from build123d import *

# Parameters (mm, degrees)
SKETCH1_W           = 8.5
SKETCH1_H           = 20
BOSS_EXTRUDE1_DEPTH = 20
SKETCH4_R           = 1
BOSS_EXTRUDE2_DEPTH = 1.5
SKETCH6_R           = 3
BOSS_EXTRUDE3_DEPTH = 3
SKETCH7_R           = 1.5
BOSS_EXTRUDE4_DEPTH = 4


with BuildPart() as part:
    # Sketch1 → Boss-Extrude1 (new body)
    with BuildSketch(Plane(origin=(0, 0, 0), x_dir=(1, 0, 0), z_dir=(0, 1, 0))):
        Rectangle(SKETCH1_W, SKETCH1_H)
    extrude(amount=BOSS_EXTRUDE1_DEPTH)

    # Sketch4 → Boss-Extrude2 (add)
    with BuildSketch(Plane(origin=(0, 15, 0), x_dir=(1, 0, 0), z_dir=(0, 1, 0))):
        Polygon((-4.25, 10), (4.25, 10), (4.25, 11.75), (2.75, 13.25), (-2.75, 13.25), (-4.25, 11.75), align=None)
        with Locations((0, 11.75)):
            Circle(SKETCH4_R, mode=Mode.SUBTRACT)
        Polygon((-2.75, -13.25), (2.75, -13.25), (4.25, -11.75), (4.25, -10), (-4.25, -10), (-4.25, -11.75), align=None)
        with Locations((0, -11.75)):
            Circle(SKETCH4_R, mode=Mode.SUBTRACT)
    extrude(amount=BOSS_EXTRUDE2_DEPTH)

    # Sketch6 → Boss-Extrude3 (add)
    with BuildSketch(Plane(origin=(0, 20, 0), x_dir=(1, 0, 0), z_dir=(0, 1, 0))):
        with Locations((0, 7)):
            Circle(SKETCH6_R)
    extrude(amount=BOSS_EXTRUDE3_DEPTH)

    # Sketch7 → Boss-Extrude4 (add)
    with BuildSketch(Plane(origin=(0, 23, 0), x_dir=(1, 0, 0), z_dir=(0, 1, 0))):
        with Locations((0, 7)):
            Circle(SKETCH7_R)
    extrude(amount=BOSS_EXTRUDE4_DEPTH)


solid = part.part
Check sheet for the modelled part. Datum: model origin and axes. Units: mm. A direction names the side the tool comes from. Give positions to 0.01 mm unless a question says otherwise; leave off trailing zeros. Loops run counter-clockwise (first coordinate to the right, second up) from the corner with the lowest first, then second, coordinate; pieces in that order, holes last. Notation, with made-up numbers: M -19.5,-35 L 23.5,-35 A15 cw 23.5,-18 Z; hole C 20.5,6.25 d8. An arc over 180 degrees is marked long. Return JSON: item names as keys, results as strings. Group by question number.
1. Cross-section at D-D on z = 6. Record the boundary of the cut face in (x, y), plus the area to 3 significant figures.
2. Cross-section at A-A on y = 16. Record the boundary of the cut face in (x, z), plus the area to 3 significant figures.
3. Mould release check, pull along X, two halves, no side actions. Record for faces 6 (the flat face through (4, 16, -12)), 7 (the cylindrical face through (-0.13, 15.74, 10.76)), 8 (the flat face through (-3, 16, -13)): released by +X, released by -X, zero draft, split by the parting line, or undercut.
4. Thickness scan on L1, parallel to Z at x = 0, y = 15.7; L2, parallel to X at y = 15.85, z = 11.75; L3, parallel to Y at x = -2.5, z = -10.5. Record the ranges inside material, lowest first.
5. Tool access check on faces 1 (the cylindrical face through (-0.325, 24.972, -5.536)), 2 (the flat face through (-1, 15, -11)), 3 (the flat face through (0, 18, 10)), 4 (the flat face through (0, 7, 10)), 5 (the flat face through (0, 18, -10)). Record the directions out of +Z, -Z, +X, -X, +Y, -Y that give a thin tool (end or side, any length) a straight path to the whole face; none if there is none.
6. Go/stop test with flat-tipped pins: pin 1 (1 mm diameter, centred on x = -1, y = 18.5, fed in from +Z); pin 2 (1.6 mm diameter, centred on x = -1, z = 11, fed in from +Y); pin 3 (3.5 mm diameter, centred on x = -1.5, z = 11, fed in from -Y); pin 4 (4 mm diameter, centred on x = -0.5, z = 0.5, fed in from +Y). Record where each tip stops, or that it passes through.
7. Cross-section at C-C on y = 5. Record the boundary of the cut face in (x, z).
8. Cross-section at B-B on z = -7. Record the boundary of the cut face in (x, y).
Return value:
{
 "1": {"outline": "M -4.25,0 L 4.25,0 L 4.25,20 L -4.25,20 Z", "area": "170 mm^2"},
 "2": {"outline": "M -4.25,-11.75 L -2.75,-13.25 L 2.75,-13.25 L 4.25,-11.75 L 4.25,11.75 L 2.75,13.25 L -2.75,13.25 L -4.25,11.75 Z; hole C 0,-11.75 d2; hole C 0,11.75 d2", "area": "214 mm^2"},
 "3": {"face 6": "released by +X", "face 7": "undercut", "face 8": "released by -X"},
 "4": {"L1": "-13.25 to -12.75, -10.75 to 10.75, 12.75 to 13.25", "L2": "-4.25 to -1, 1 to 4.25", "L3": "15 to 16.5"},
 "5": {"face 1": "+Y", "face 2": "-Z, +X, -X, -Y", "face 3": "+Z, +X, -X, +Y", "face 4": "+Z, +X, -X, -Y", "face 5": "-Z, +X, -X, +Y"},
 "6": {"pin 1": "z = 10", "pin 2": "y = 16.5", "pin 3": "y = 0", "pin 4": "y = 20"},
 "7": {"outline": "M -4.25,-10 L 4.25,-10 L 4.25,10 L -4.25,10 Z"},
 "8": {"outline": "M -4.25,0 L 4.25,0 L 4.25,20 L 3,20 L 3,23 L 1.5,23 L 1.5,27 L -1.5,27 L -1.5,23 L -3,23 L -3,20 L -4.25,20 Z"}
}
